```python
from build123d import *

# Parameters (mm, degrees)
F0_W     = 70.120454
F0_H     = 10.372847
F0_H_2   = 14.521986
F1_DEPTH = 12.7
F2_DEPTH = 12.7
F4_D     = 12.7


with BuildPart() as f1:
    # F0 (on Top) → F1 (new body)
    with BuildSketch(Plane.XY):
        with Locations((0, -12.447416)):
            Rectangle(F0_W, F0_H)
        Rectangle(F0_W, F0_H_2)
        with Locations((0, 12.447416)):
            Rectangle(F0_W, F0_H)
    extrude(amount=-F1_DEPTH)

    # F0 (on Top) → F2 (join)
    with BuildSketch(Plane.XY):
        Rectangle(F0_W, F0_H_2)
    extrude(amount=F2_DEPTH)

    # F4 (through all)
    with Locations(Plane.XY.offset(12.7)):
        with Locations((0, 0)):
            Hole(F4_D / 2)


solid = f1.part
```
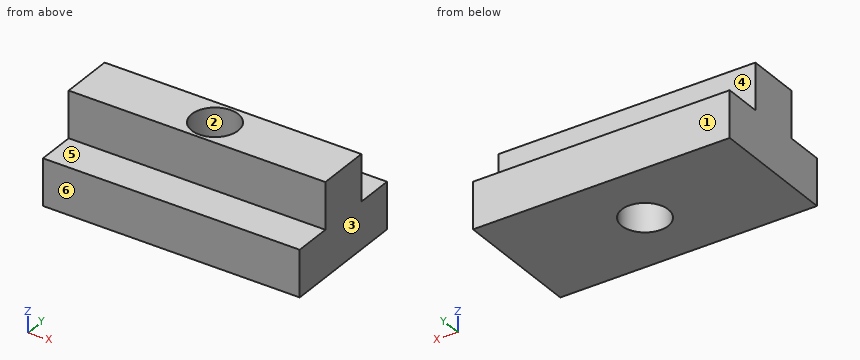
Design review of the part built by this model. Coordinates are the model's own, in mm. Face numbers are marked on the shaded views. A direction names the side the tool comes from. Coordinates: 2 decimals unless noted, no trailing zeros. Write each loop counter-clockwise with the first axis right and the second up, starting at its lowest first coordinate (ties: lowest second). Pieces come first, ordered by that corner, then holes. Notation, with made-up numbers: M -8.5,64 L 13.5,64 A14 ccw 13.5,89 Z; hole C 3,-13.5 d4. An arc over 180 degrees is marked long. Answer as a JSON object with one key per item and string values.
Item 1: Add section A-A, the plane y = 0. Give the boundary of the cut face in (x, z), and give its area (3 significant figures).
Outcome:
{"outline": "M -35.06,-12.7 L -6.35,-12.7 L -6.35,12.7 L -35.06,12.7 Z; M 6.35,-12.7 L 35.06,-12.7 L 35.06,12.7 L 6.35,12.7 Z", "area": "1,460 mm²"}
Item 2: Draft analysis for pull direction Y (two halves, no side actions). For the marked faces 1, 2 and 3, state which applies: pulls with the +Y half, pulls with the -Y half, needs draft (parallel to the pull), parting line crosses it, or undercut.
Outcome:
{"face 1": "pulls with the +Y half", "face 2": "undercut", "face 3": "needs draft"}
Item 3: Wall thickness on probe 1 along Y at (x, z) = (0, 5.75); probe 2 along Y at (x, z) = (8.5, 2.5); probe 3 along Z at (x, y) = (0.5, 7.5): over which ranges is each line inside the solid? List them lowest first.
Outcome:
{"probe 1": "-7.26 to -6.35, 6.35 to 7.26", "probe 2": "-7.26 to 7.26", "probe 3": "-12.7 to 0"}
Item 4: Machinability: for the marked faces 4, 5 and 6, which of the approach directions +Z, -Z, +X, -X, +Y, -Y give a long, thin tool a straight path to every point of the face, cutting with its end or side? Answer none if there is none.
Outcome:
{"face 4": "+Z, +X, -X, +Y", "face 5": "+Z, +X, -X, -Y", "face 6": "+Z, -Z, +X, -X, -Y"}
Item 5: Add section D-D, the plane x = 12.5. Give the boundary of the cut face in (y, z), and give its area (3 significant figures).
Outcome:
{"outline": "M -17.63,-12.7 L 17.63,-12.7 L 17.63,0 L 7.26,0 L 7.26,12.7 L -7.26,12.7 L -7.26,0 L -17.63,0 Z", "area": "632 mm²"}
Item 6: Add section C-C, the plane z = -5.5. Give the boundary of the cut face in (x, y), and give its area (3 significant figures).
Outcome:
{"outline": "M -35.06,-17.63 L 35.06,-17.63 L 35.06,17.63 L -35.06,17.63 Z; hole C 0,0 d12.7", "area": "2,350 mm²"}
Item 7: Insertion check: pin 1 Ø4 at (x, z) = (1.5, 8) entering from +Y; pin 2 Ø3 at (x, y) = (-0.5, 13.5) entering from +Z; pin 3 Ø4 at (x, z) = (-15.5, 4) entering from -Y. Each pin has a flat end and moves straight along its axis. Give the tip position at first contact, or say it passes through.
Outcome:
{"pin 1": "y = 7.26", "pin 2": "z = 0", "pin 3": "y = -7.26"}
Item 8: Add section B-B, the plane x = 0. Give the boundary of the cut face in (y, z), and give its area (3 significant figures).
Outcome:
{"outline": "M -17.63,-12.7 L -6.35,-12.7 L -6.35,12.7 L -7.26,12.7 L -7.26,0 L -17.63,0 Z; M 6.35,-12.7 L 17.63,-12.7 L 17.63,0 L 7.26,0 L 7.26,12.7 L 6.35,12.7 Z", "area": "310 mm²"}
